Autodesk Inventor part; units mm, degrees
ref_plane "YZ Plane" through (0, 0, 0) normal (1, 0, 0) x (0, 1, 0)
ref_plane "XZ Plane" through (0, 0, 0) normal (0, 1, 0) x (-1, 0, 0)
ref_plane "XY Plane" through (0, 0, 0) normal (0, 0, 1) x (1, 0, 0)
sketch "Sketch1" plane through (0, 0, 0) normal (0, 0, 1) x (1, 0, 0)
  circle A0 centre (3.25, 6.65) radius 1.2295
  line L0 (0, 0) -> (6.5, 0)
  line L1 (6.5, 0) -> (6.5, 9.3)
  line L2 (6.5, 9.3) -> (0, 9.3)
  line L3 (0, 0) -> (0, 9.3)
  circle A1 centre (3.25, 13.15) radius 1.2295
  line L4 (0, 9.3) -> (6.5, 9.3)
  line L5 (6.5, 9.3) -> (6.5, 17)
  line L6 (0, 17) -> (6.5, 17)
  line L7 (0, 9.3) -> (0, 17)
  circle A2 centre (3.25, -45.05) radius 1.2295
  line L8 (0.5983, -42.4) -> (0, -42.4)
  line L9 (0, -42.4) -> (0, -47.7)
  line L10 (0, -47.7) -> (6.5, -47.7)
  line L11 (6.5, -38.4) -> (6.5, -47.7)
  line L12 (0.5983, -38.4) -> (6.5, -38.4)
  line L13 (0.5983, -38.4) -> (0.5983, -42.4)
  circle A3 centre (3.25, -51.55) radius 1.2295
  line L14 (0, -47.7) -> (6.5, -47.7)
  line L15 (0, -47.7) -> (0, -55.4)
  line L16 (6.5, -55.4) -> (0, -55.4)
  line L17 (6.5, -47.7) -> (6.5, -55.4)
  circle A4 centre (-9.75, -51.55) radius 1.2295
  line L18 (-41.3371, -47.7) -> (-6.5, -47.7)
  line L19 (-41.3371, -47.7) -> (-41.3371, -49.7)
  line L20 (-13, -49.7) -> (-41.3371, -49.7)
  line L21 (-13, -49.7) -> (-13, -55.4)
  line L22 (-6.5, -55.4) -> (-13, -55.4)
  line L23 (-6.5, -47.7) -> (-6.5, -55.4)
  circle A5 centre (-9.75, 13.15) radius 1.2295
  line L24 (-41.3371, 11.3) -> (-13, 11.3)
  line L25 (-41.3371, 9.3) -> (-41.3371, 11.3)
  line L26 (-41.3371, 9.3) -> (-6.5, 9.3)
  line L27 (-6.5, 9.3) -> (-6.5, 17)
  line L28 (-13, 17) -> (-6.5, 17)
  line L29 (-13, 11.3) -> (-13, 17)
  arc A6 (-64.7971, 16.2257) -> (-64.1621, 16.7072) centre (-64.6621, 16.7072) ccw
  line L30 (-64.1621, 16.7072) -> (-64.1621, 23.8)
  arc A7 (-64.1621, 23.8) -> (-67.1621, 26.8) centre (-67.1621, 23.8) ccw
  line L31 (-67.1621, 26.8) -> (-70.1621, 26.8)
  line L32 (-70.1621, 26.8) -> (-70.1621, 29.3)
  line L33 (-70.1621, 29.3) -> (-59.3371, 29.3)
  line L34 (-59.3371, 29.3) -> (-59.3371, 30.8)
  line L35 (-59.3371, 30.8) -> (-78.8451, 30.8)
  line L36 (-78.8451, 16.3) -> (-78.8451, 30.8)
  line L37 (-65.3371, 16.3) -> (-78.8451, 16.3)
  arc A8 (-64.7971, 16.2257) -> (-65.3371, 16.3) centre (-65.3371, 14.3) ccw
  circle A9 centre (-67.4121, 21.8) radius 1.2295
  circle A10 centre (-74.1621, 21.8) radius 1.2295
  circle A11 centre (-67.4121, -60.2) radius 1.2295
  circle A12 centre (-74.1621, -60.2) radius 1.2295
  arc A13 (-64.1621, -55.1072) -> (-64.7971, -54.6257) centre (-64.6621, -55.1072) ccw
  arc A14 (-65.3371, -54.7) -> (-64.7971, -54.6257) centre (-65.3371, -52.7) ccw
  line L38 (-65.3371, -54.7) -> (-78.8451, -54.7)
  line L39 (-78.8451, -54.7) -> (-78.8451, -69.2)
  line L40 (-59.3371, -69.2) -> (-78.8451, -69.2)
  line L41 (-59.3371, -67.7) -> (-59.3371, -69.2)
  line L42 (-59.3371, -67.7) -> (-70.1621, -67.7)
  line L43 (-70.1621, -67.7) -> (-70.1621, -65.2)
  line L44 (-70.1621, -65.2) -> (-67.1621, -65.2)
  arc A15 (-67.1621, -65.2) -> (-64.1621, -62.2) centre (-67.1621, -62.2) ccw
  line L45 (-64.1621, -62.2) -> (-64.1621, -55.1072)
  line L46 (-59.3371, 30.8) -> (-59.3371, 11.3)
  line L47 (-59.3371, 11.3) -> (-41.3371, 11.3)
  line L48 (-41.3371, 9.3) -> (-76.8451, 9.3)
  line L49 (-78.8451, 16.3) -> (-78.8451, -54.7)
  line L50 (-76.8451, 9.3) -> (-76.8451, -47.7)
  line L51 (-76.8451, -47.7) -> (-41.3371, -47.7)
  line L52 (-41.3371, -49.7) -> (-59.3371, -49.7)
  line L53 (-59.3371, -49.7) -> (-59.3371, -67.7)
  line L54 (-6.5, 17) -> (0, 17)
  line L55 (-6.5, 9.3) -> (0, 9.3)
  line L56 (-6.5, -47.7) -> (0, -47.7)
  line L57 (-6.5, -55.4) -> (0, -55.4)
  line L58 (6.5, 0) -> (6.5, -38.4)
  line L59 (4.5, -38.4) -> (4.5, 0)
  dimension "d0" = 2
  dimension "d1" = 2
extrude "Extrusion1" add sketch "Sketch1" along normal blind 2 contours L3 L2 L1 L0 | L0 L58 L12 L59 | L7 L6 L5 L2 | L55 L27 L54 L7 | L12 L11 L10 L9 L8 L13 | L26 L25 L24 L29 L28 L27 | L48 L50 L51 L19 L52 L53 L42 L43 L44 A15 L45 A13 A14 L38 L49 L37 A8 A6 L30 A7 L31 L32 L33 L46 L47 L25 | L17 L16 L15 L10 | L15 L57 L23 L56 | L23 L22 L21 L20 L19 L18 | L33 L32 L31 A7 L30 A6 A8 L37 L36 L35 L34 | L41 L40 L39 L38 A14 A13 L45 A15 L44 L43 L42
fillet "Fillet1" radius 2 10 edges at (-76.8451, 9.3, 1) (-76.8451, -47.7, 1) (0.5983, -42.4, 1) (0, -42.4, 1) (0.5983, -38.4, 1) (4.5, -38.4, 1) (0, -47.7, 1) (0, 9.3, 1) (0, 0, 1) (4.5, 0, 1)
properties part number "CeilUphold"
CAD build for the part. Positions are in the model's coordinates, mm. A direction names the side the tool comes from. Coordinates: 2 decimals unless noted, no trailing zeros. Order: outer loops, then holes, each group sorted by start corner. A loop starts at its lowest first (then second) coordinate and runs counter-clockwise, first axis right, second up. Notation, with made-up numbers: (-30.75, 44) - (-10.75, 44) arc R19 cw to (-10.75, 62) - close; hole circle Ø2 at (-31, -29). An arc over 180 degrees is marked (long way). Use a Markdown table: item, result. Add a question column.
(1) Saw through at C-C (y = 13.15). Give the cut face in (x, z), then the cut area to 3 significant figures.
(2) Flat gauge pins, fed straight in: pin 1 (1 mm diameter, centred on x = -43, z = 1, fed in from +Y); pin 2 (1.5 mm diameter, centred on x = 3.25, y = 13.15, fed in from +Z); pin 3 (0.6 mm diameter, centred on x = -23, z = 1, fed in from -Y); pin 4 (0.6 mm diameter, centred on x = -1.5, z = 1, fed in from -Y). Where does each tip first touch, or does it go through?
(3) Pull direction Y, two halves, no side cores. Call faces 4 (the face through (-3, 17, 1)), 5 (the face through (-0.6, 8.73, 0.99)), 6 (the face through (6.5, -20, 1)), 7 (the face through (-39, -47.7, 1)): +Y half, -Y half, draft (parallel to the pull), parting line (faces both ways), or undercut.
(4) Saw through at B-B (x = -16). Give the cut face in (y, z), then the cut area to 3 significant figures.
(5) Saw through at A-A (y = -16.5). Give the cut face in (x, z), then the cut area to 3 significant figures.
(6) Saw through at D-D (z = 1.25). Count the separate pieces of the cut face and the enclosed holes in it, then the cut area to 3 significant figures.
(7) Which spindle directions (+Z, -Z, +X, -X, +Y, -Y) get a long thin tool onto all of the face, cutting with end or side? Do faces 1 (the face through (-69, 30.8, 1)), 2 (the face through (-59.337, -59, 1)), 3 (the face through (-39, 9.3, 1)). Say none if no direction does.
(8) Drill centre lines: line 1 along Y through (x, z) = (-59.5, 1.75); line 2 along Y through (x, z) = (-42, 0.45); line 3 along X through (y, z) = (15, 0.6). Where is each one in solid material? Low to high. Write a range as [from, to].
Solved:
| question | item | result |
|---|---|---|
| 1 | outline | (-78.85, 0) - (-59.34, 0) - (-59.34, 2) - (-78.85, 2) - close; (-13, 0) - (-10.98, 0) - (-10.98, 2) - (-13, 2) - close; (-8.52, 0) - (2.02, 0) - (2.02, 2) - (-8.52, 2) - close; (4.48, 0) - (6.5, 0) - (6.5, 2) - (4.48, 2) - close |
| 1 | area | 68.2 mm² |
| 2 | pin 1 | stops at y = 11.3 |
| 2 | pin 2 | passes through |
| 2 | pin 3 | stops at y = -49.7 |
| 2 | pin 4 | stops at y = -55.4 |
| 3 | face 4 | +Y half |
| 3 | face 5 | undercut |
| 3 | face 6 | draft |
| 3 | face 7 | undercut |
| 4 | outline | (-49.7, 0) - (-47.7, 0) - (-47.7, 2) - (-49.7, 2) - close; (9.3, 0) - (11.3, 0) - (11.3, 2) - (9.3, 2) - close |
| 4 | area | 8.00 mm² |
| 5 | outline | (-78.85, 0) - (-76.85, 0) - (-76.85, 2) - (-78.85, 2) - close; (4.5, 0) - (6.5, 0) - (6.5, 2) - (4.5, 2) - close |
| 5 | area | 8.00 mm² |
| 6 | separate pieces | 1 |
| 6 | enclosed holes | 11 |
| 6 | area | 1,590 mm² |
| 7 | face 1 | +Z, -Z, +X, -X, +Y |
| 7 | face 2 | +Z, -Z, -Y |
| 7 | face 3 | +Z, -Z |
| 8 | line 1 | y = [-69.2, -47.7], [9.3, 30.8] |
| 8 | line 2 | y = [-49.7, -47.7], [9.3, 11.3] |
| 8 | line 3 | x = [-78.85, -59.34], [-13, 6.5] |
